CAD build for the part. Positions are in the model's coordinates, mm. A direction names the side the tool comes from. Coordinates: 2 decimals unless noted, no trailing zeros. Order: outer loops, then holes, each group sorted by start corner. A loop starts at its lowest first (then second) coordinate and runs counter-clockwise, first axis right, second up. Notation, with made-up numbers: M -35.5,18.5 L -25.5,18.5 A20 cw -25.5,42.5 Z; hole C 46.5,-26 d3. An arc over 180 degrees is marked long. Write item = value, one per line.
from build123d import *

# Parameters (mm, degrees)
F1_DEPTH = 63.5
F2_DEPTH = 25.4
F3_DEPTH = 15.875
F0_W     = 18.50829
F0_H     = 19.05
F5_R     = 6.35


with BuildPart() as f1:
    # F0 (on Front) → F1 (new body, symmetric)
    with BuildSketch(Plane.XZ):
        Polygon((41.275, -9.525), (41.275, 9.525), (22.225, 9.525), (-41.275, 9.525), (-41.275, -9.525), align=None)
    extrude(amount=F1_DEPTH, both=True)

    # F0 (on Front) → F2 (join, symmetric)
    with BuildSketch(Plane.XZ):
        with BuildLine():
            Line((22.225, 9.525), (41.275, 9.525))
            Line((41.275, 9.525), (41.275, 27.0002))
            ThreePointArc((41.275, 27.0002), (45.92468, 38.22552), (57.15, 42.8752))
            Line((57.15, 42.8752), (60.325, 42.8752))
            Line((60.325, 42.8752), (60.325, 61.9252))
            Line((60.325, 61.9252), (57.15, 61.9252))
            add(Edge.make_bspline(
                [(56.529617, 61.91969), (56.73609, 61.921736), (56.942884, 61.923573), (57.15, 61.9252)],
                knots=[111.11806, 111.11806, 111.11806, 111.11806, 111.504536, 111.504536, 111.504536, 111.504536], degree=3))
            ThreePointArc((56.529617, 61.91969), (32.235922, 51.475583), (22.225, 27.0002))
            Line((22.225, 27.0002), (22.225, 9.525))
        make_face()
    extrude(amount=F2_DEPTH, both=True)

    # F0 (on Front) → F3 (join)
    with BuildSketch(Plane.XZ):
        with BuildLine():
            Line((-41.275, 9.525), (22.225, 9.525))
            Line((22.225, 9.525), (22.225, 27.0002))
            ThreePointArc((22.225, 27.0002), (32.235922, 51.475583), (56.529617, 61.91969))
            add(Edge.make_bspline(
                [(-41.275, 9.525), (-35.629907, 43.413288), (-2.834722, 61.331295), (56.529617, 61.91969)],
                knots=[0, 0, 0, 0, 111.11806, 111.11806, 111.11806, 111.11806], degree=3))
        make_face()
    extrude(amount=F3_DEPTH)

    # F0 (on Front) → F4 (revolve)
    with BuildSketch(Plane.XZ):
        with Locations((69.579145, 52.4002)):
            Rectangle(F0_W, F0_H)
    revolve(axis=Axis((60.325, 0, 52.3875), (0, 0, 1)))

    # F5
    f5_edges = [f1.edges().sort_by_distance(p)[0] for p in [
        (41.275, -63.5, 0),
        (-41.275, -63.5, 0),
        (41.275, 63.5, 0),
        (-41.275, 63.5, 0),
    ]]
    fillet(f5_edges, radius=F5_R)


solid = f1.part
(1) Slice it at A-A, the plane z = 4.5. Write the cut outline in (x, y) (3 decimals).
Evaluation:
outline = M -41.275,-57.15 A6.35 ccw -34.925,-63.5 L 34.925,-63.5 A6.35 ccw 41.275,-57.15 L 41.275,57.15 A6.35 ccw 34.925,63.5 L -34.925,63.5 A6.35 ccw -41.275,57.15 Z
(2) Tool access for faces 1 (the face through (22.225, 13, 18)), 2 (the face through (37, 25.4, 36)), 3 (the face through (22.225, -21, 18)), 4 (the face through (41.275, -1, 4)): list every direction of +Z, -Z, +X, -X, +Y, -Y with a clear straight run to the whole face (end or side of a thin tool).
Evaluation:
face_1 = +Z, -X, +Y
face_2 = +Z, +X, -X, +Y
face_3 = +Z, -X, -Y
face_4 = -Z, +X, +Y, -Y
(3) Wall check: line 1 (X direction, y = 28, z = -5.5) (3 decimals); line 2 (Z direction, x = 38.5, y = 51) (3 decimals); line 3 (Y direction, x = 41, z = 47). Give the ranges that are in metal, low to high. Write a range as from..to.
Evaluation:
line_1 = -41.275..41.275
line_2 = -9.525..9.525
line_3 = -25.4..25.4
(4) Pin check, flat tips, straight feed: pin 1 Ø1.5 at (y, z) = (-3.5, 48.5) entering from +X; pin 2 Ø5 at (y, z) = (17.5, 21) entering from -X (3 decimals); pin 3 Ø3.5 at (y, z) = (-21.5, 53.5) entering from +X (3 decimals); pin 4 Ø2 at (x, y) = (62, 27.5) entering from +Z. Stop position of each tip, or through.
Evaluation:
pin_1 = 78.63
pin_2 = 22.225
pin_3 = 60.325
pin_4 = through
(5) Slice it at B-B, the plane y = -51. Write the cut outline in (x, z) (3 decimals).
Evaluation:
outline = M -41.275,-9.525 L 41.275,-9.525 L 41.275,9.525 L -41.275,9.525 Z
